from build123d import *

# Parameters (mm, degrees)
SKETCH1_R                = 4.50864138
SKETCH1_R_2              = 2
SKETCH1_R_3              = 4.6
SKETCH1_R_4              = 1.429414062
BOSS_EXTRUDE1_DEPTH      = 3.175
SKETCH2_W                = 597.466303312
SKETCH2_H                = 60.972543052
CUT_EXTRUDE1_DEPTH       = 70
FILLET1_R                = 10
FILLET2_R                = 10
SKETCH6_R                = 40
BOSS_EXTRUDE2_DEPTH      = 3.175
BOSS_EXTRUDE3_DEPTH      = 3.175
SKETCH9_R                = 40
BOSS_EXTRUDE4_DEPTH      = 3.175
BOSS_EXTRUDE6_DEPTH      = 3.175
SKETCH13_R               = 19
CUT_EXTRUDE5_DEPTH       = 10
SKETCH14_R               = 19
CUT_EXTRUDE6_DEPTH       = 10
BOSS_EXTRUDE7_DEPTH      = 10
BOSS_EXTRUDE7_DEPTH_BACK = 3.175
SKETCH16_W               = 39.380598922
SKETCH16_H               = 33.904845405
CUT_EXTRUDE7_DEPTH       = 10


with BuildPart() as part:
    # Sketch1 → Boss-Extrude1 (new body)
    with BuildSketch(Plane(origin=(0, 0, 0), x_dir=(1, 0, 0), z_dir=(0, 1, 0))):
        with BuildLine():
            ThreePointArc((8, 150), (2.343145751, 147.656854249), (0, 142))
            Line((0, 142), (42, 8))
            ThreePointArc((42, 8), (44.343145751, 2.343145751), (50, 0))
            Line((50, 0), (436.5, 0))
            ThreePointArc((436.5, 0), (442.156854249, 2.343145751), (444.5, 8))
            Line((444.5, 8), (444.5, 142))
            ThreePointArc((444.5, 142), (442.156854249, 147.656854249), (436.5, 150))
            Line((436.5, 150), (338.059360585, 150))
            ThreePointArc((338.059360585, 150), (334.223325972, 144.782574379), (330.387291359, 150))
            Line((330.387291359, 150), (282.940349401, 150))
            ThreePointArc((282.940349401, 150), (281.106475607, 148.798064477), (279.272601814, 150))
            Line((279.272601814, 150), (172.868406334, 150))
            ThreePointArc((172.868406334, 150), (172.5, 146.64039861), (172.131593666, 150))
            Line((172.131593666, 150), (123.116119719, 150))
            ThreePointArc((123.116119719, 150), (122, 146.34039861), (120.883880281, 150))
            Line((120.883880281, 150), (8, 150))
        make_face()
        with Locations(Location((182.429479385, 77.355745695, 0), (0, 0, 270))):
            Circle(SKETCH1_R, mode=Mode.SUBTRACT)
        with Locations(Location((388.475756445, 100.077126905, 0), (0, 0, 270))):
            Circle(SKETCH1_R_2, mode=Mode.SUBTRACT)
        with Locations(Location((265.281257274, 74.563866981, 0), (0, 0, 270))):
            Circle(SKETCH1_R_3, mode=Mode.SUBTRACT)
        with Locations(Location((25.854352659, 89.089252974, 0), (0, 0, 270))):
            Circle(SKETCH1_R_4, mode=Mode.SUBTRACT)
        with Locations(Location((77.821750814, 98.327219393, 0), (0, 0, 270))):
            Circle(SKETCH1_R_2, mode=Mode.SUBTRACT)
    extrude(amount=BOSS_EXTRUDE1_DEPTH)

    # Sketch2 → Cut-Extrude1 (cut)
    with BuildSketch(Plane.XY):
        with Locations((220.1785332, 7.544358636)):
            Rectangle(SKETCH2_W, SKETCH2_H)
    extrude(amount=-CUT_EXTRUDE1_DEPTH, mode=Mode.SUBTRACT)

    # Fillet1
    fillet1_edges = [part.edges().sort_by_distance(p)[0] for p in [
        (22.567164179, 1.5875, -70),
    ]]
    fillet(fillet1_edges, radius=FILLET1_R)

    # Fillet2
    fillet2_edges = [part.edges().sort_by_distance(p)[0] for p in [
        (444.5, 1.5875, -70),
    ]]
    fillet(fillet2_edges, radius=FILLET2_R)

    # Sketch6 → Boss-Extrude2 (add)
    with BuildSketch(Plane(origin=(0, 0, 0), x_dir=(1, 0, 0), z_dir=(0, 1, 0))):
        with Locations((149, 150.04039861)):
            Circle(SKETCH6_R)
    extrude(amount=BOSS_EXTRUDE2_DEPTH)

    # Sketch7 → Boss-Extrude3 (add)
    with BuildSketch(Plane(origin=(0, 0, 0), x_dir=(1, 0, 0), z_dir=(0, 1, 0))):
        Polygon((124.164543783, 181.396420591), (82.702881078, 149.750534228), (231.468946681, 149.750534228), (173.835456217, 181.396420591), align=None)
    extrude(amount=BOSS_EXTRUDE3_DEPTH)

    # Sketch9 → Boss-Extrude4 (add)
    with BuildSketch(Plane(origin=(0, 0, 0), x_dir=(1, 0, 0), z_dir=(0, 1, 0))):
        with BuildLine():
            ThreePointArc((269, 150), (272.870833001, 167.166341835), (283.734164599, 181.010281545))
            Line((283.734164599, 181.010281545), (245.673378314, 150))
            Line((245.673378314, 150), (269, 150))
        make_face()
        with Locations((309, 150)):
            Circle(SKETCH9_R)
    extrude(amount=BOSS_EXTRUDE4_DEPTH)

    # Sketch12 → Boss-Extrude6 (add)
    with BuildSketch(Plane(origin=(0, 0, 0), x_dir=(1, 0, 0), z_dir=(0, 1, 0))):
        Polygon((326.166341835, 186.129166999), (382.106475607, 150), (340.398839744, 150), align=None)
    extrude(amount=BOSS_EXTRUDE6_DEPTH)

    # Sketch13 → Cut-Extrude5 (cut)
    with BuildSketch(Plane(origin=(0, 3.175, 0), x_dir=(1, 0, 0), z_dir=(0, 1, 0))):
        with Locations(Location((146, 139.84039861, 0), (0, 0, 270))):
            Circle(SKETCH13_R)
    extrude(amount=-CUT_EXTRUDE5_DEPTH, mode=Mode.SUBTRACT)

    # Sketch14 → Cut-Extrude6 (cut)
    with BuildSketch(Plane(origin=(0, 3.175, 0), x_dir=(1, 0, 0), z_dir=(0, 1, 0))):
        with Locations(Location((307.606475607, 142.298064477, 0), (0, 0, 270))):
            Circle(SKETCH14_R)
    extrude(amount=-CUT_EXTRUDE6_DEPTH, mode=Mode.SUBTRACT)

    # Sketch15 → Boss-Extrude7 (add, two sides: drawn at the far end of the back side and taken through both)
    with BuildSketch(Plane(origin=(0, 3.175, 0), x_dir=(1, 0, 0), z_dir=(0, 1, 0)).offset(-BOSS_EXTRUDE7_DEPTH_BACK)):
        with BuildLine():
            Line((270.323640372, 61.870718801), (281.671389991, 70))
            Line((281.671389991, 70), (265.856685963, 70))
            ThreePointArc((265.856685963, 70), (269.551101507, 72.852601302), (268.849345077, 77.467097842))
            Line((268.849345077, 77.467097842), (266.045546336, 79.099929396))
            ThreePointArc((266.045546336, 79.099929396), (260.730312777, 75.233870106), (264.705828584, 70))
            Line((264.705828584, 70), (252.589726142, 70))
            Line((252.589726142, 70), (257.164027826, 63.204154779))
            ThreePointArc((257.164027826, 63.204154779), (263.491883069, 60.050944756), (270.323640372, 61.870718801))
        make_face()
    extrude(amount=BOSS_EXTRUDE7_DEPTH + BOSS_EXTRUDE7_DEPTH_BACK)

    # Sketch16 → Cut-Extrude7 (cut)
    with BuildSketch(Plane(origin=(0, 13.175, 0), x_dir=(1, 0, 0), z_dir=(0, 1, 0))):
        with Locations((267.135263248, 68.050551455)):
            Rectangle(SKETCH16_W, SKETCH16_H)
    extrude(amount=-CUT_EXTRUDE7_DEPTH, mode=Mode.SUBTRACT)


solid = part.part
Geometry: final body of the model. Coordinates: model frame, mm. A direction names the side the tool comes from. Round coordinates to 2 decimals unless told otherwise and drop trailing zeros. Order: outer loops, then holes, each group sorted by start corner. A loop starts at its lowest first (then second) coordinate and runs counter-clockwise, first axis right, second up. Notation, with made-up numbers: (56, 3.5) -> (62, 3.5) arc R26 ccw to (62, 23.5) -> close; hole circle Ø5 at (-9, 51.5). An arc over 180 degrees is marked (long way). Put each result on its own line as item: value. Start each with the question number.
Q1. Reachability of faces 4 (the flat face through (358.158, 1.565, -165.467)), 5 (the flat face through (202.825, 1.565, -165.478)) from +Z, -Z, +X, -X, +Y, -Y: full face, straight path, thin tool, end or side. Return the list, or none.
Q2. Section C-C on z = -107.5. Return the cut outline in (x, y) (3 decimals).
Q3. Line query: probe 1 along X at (y, z) = (0.55, -146.5); probe 2 along X at (y, z) = (0.9, -146); probe 3 along X at (y, z) = (3.05, -151.5). Output: solid intervals per line, ascending.
Q4. First-contact query: pin 1 (7 mm diameter, centred on x = 182.43, z = -77.36, fed in from +Y); pin 2 (1.6 mm diameter, centred on x = 397, y = 2.5, fed in from -Z); pin 3 (1 mm diameter, centred on x = 360, y = 1.5, fed in from +Z). Flat tips, straight axial feed; report the tip coordinate or a pass-through.
Q5. Pull-direction query (X, two-part tool) for faces 1 (the cylindrical face through (186.9, 1.57, -77.94)), 2 (the cylindrical face through (2.406, 1.565, -147.719)), 3 (the flat face through (219, 0, -126)); classes: +X half, -X half, draft (parallel to the pull), parting line (faces both ways), or undercut.
Q6. Section A-A on x = 146. Return the cut outline in (y, z) (3 decimals), and give its area (3 significant figures).
Q7. Section B-B on y = 2.4. Return the cut outline in (x, z).
Ans:
1. face 4: -Z, +X, +Y, -Y
1. face 5: -Z, +Y, -Y
2. outline: (10.813, 0) -> (444.5, 0) -> (444.5, 3.175) -> (10.813, 3.175) -> close
3. probe 1: x = 1.39 to 128.21, 163.79 to 289.08, 326.14 to 443.11
3. probe 2: x = 1.07 to 128.03, 163.97 to 288.97, 326.24 to 443.43
3. probe 3: x = 84.99 to 131, 161 to 228.28, 247.51 to 290.98, 324.23 to 379.78
4. pin 1: passes through
4. pin 2: stops at z = -150
4. pin 3: stops at z = -70
5. face 1: undercut
5. face 2: -X half
5. face 3: draft
6. outline: (0, -189.928) -> (3.175, -189.928) -> (3.175, -158.84) -> (0, -158.84) -> close; (0, -120.84) -> (3.175, -120.84) -> (3.175, -70) -> (0, -70) -> close
6. area: 260 mm2
7. outline: (0, -142) arc R8 ccw to (8, -150) -> (83.03, -150) -> (124.16, -181.4) arc R40 ccw to (173.84, -181.4) -> (231.01, -150) -> (245.67, -150) -> (283.73, -181.01) arc R40 ccw to (334.87, -180.51) -> (382.11, -150) -> (436.5, -150) arc R8 ccw to (444.5, -142) -> (444.5, -80) arc R10 ccw to (434.5, -70) -> (281.67, -70) -> (270.32, -61.87) arc R10 ccw to (257.16, -63.2) -> (252.59, -70) -> (29.91, -70) arc R10 ccw to (20.37, -77.01) -> close; hole circle Ø2.86 at (25.85, -89.09); hole circle Ø4 at (77.82, -98.33); hole circle Ø38 at (146, -139.84); hole circle Ø9.02 at (182.43, -77.36); hole (266.05, -79.1) arc R4.6 ccw to (268.85, -77.47) -> close; hole circle Ø38 at (307.61, -142.3); hole circle Ø4 at (388.48, -100.08)
